Drawing for the job (mm, zero at the part's lowest x, y, z). A direction names the side the tool comes from. Round coordinates to 2 decimals unless told otherwise and drop trailing zeros. Write each loop counter-clockwise with the first axis right and the second up, starting at its lowest first coordinate (ties: lowest second). Pieces come first, ordered by that corner, then holes. Notation, with made-up numbers: (38.5, 85.5) - (75.5, 85.5) arc R11 ccw to (75.5, 95.5) - close; hole circle Ø4 at (89, 39). An arc over 180 degrees is marked (long way). Answer in a Markdown table with one row per item.
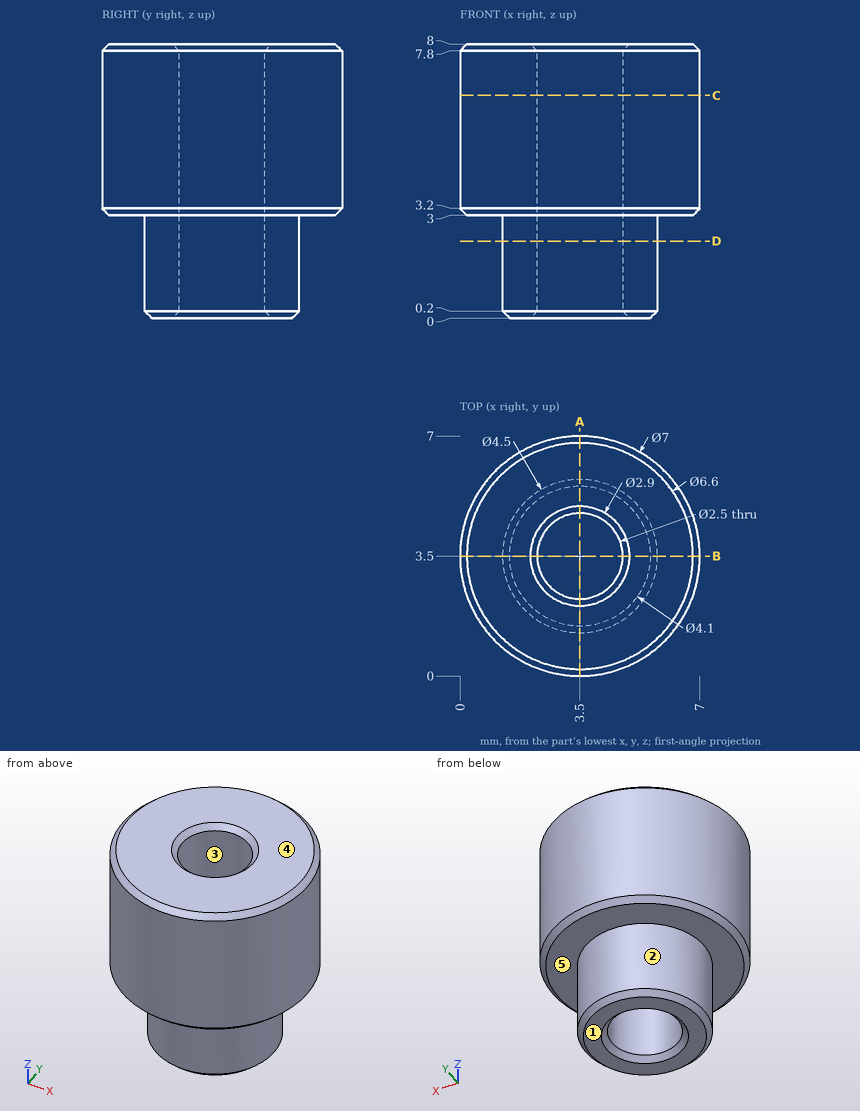
Q1. Saw through at A-A on x = 3.5. List the corners of the cut face in (y, z), then the cut area to 3 significant figures.
Computed:
| item | result |
|---|---|
| outline | (0, 3.2) - (0.2, 3) - (1.25, 3) - (1.25, 0.2) - (1.45, 0) - (2.05, 0) - (2.25, 0.2) - (2.25, 7.8) - (2.05, 8) - (0.2, 8) - (0, 7.8) - close; (4.75, 0.2) - (4.95, 0) - (5.55, 0) - (5.75, 0.2) - (5.75, 3) - (6.8, 3) - (7, 3.2) - (7, 7.8) - (6.8, 8) - (4.95, 8) - (4.75, 7.8) - close |
| area | 28.3 mm2 |
Q2. Drill centre lines: line 1 (Y direction, x = 3.5, z = 6); line 2 (Y direction, x = 3.5, z = 2); line 3 (Z direction, x = 5.75, y = 1.75). Where is each one in solid material? Low to high.
Computed:
| item | result |
|---|---|
| line 1 | y = 0 to 2.25, 4.75 to 7 |
| line 2 | y = 1.25 to 2.25, 4.75 to 5.75 |
| line 3 | z = 3 to 8 |
Q3. Pull direction Y, two halves, no side cores. Call the marked faces 1, 2 and 3: released by +Y, released by -Y, zero draft, split by the parting line, or undercut.
Computed:
| item | result |
|---|---|
| face 1 | zero draft |
| face 2 | split by the parting line |
| face 3 | undercut |
Q4. 3-axis set-ups, long thin cutter, end or side, ignore diameter. For the marked faces 4 and 5: which of +Z, -Z, +X, -X, +Y, -Y reach the whole face in a straight line?
Computed:
| item | result |
|---|---|
| face 4 | +Z, +X, -X, +Y, -Y |
| face 5 | -Z |
Q5. Flat gauge pin, fed straight in: pin 1 (2 mm diameter, centred on y = 5.5, z = 3, fed in from -X). Where does the tip first touch, or does it go through?
Computed:
| item | result |
|---|---|
| pin 1 | stops at x = 0.15 |
Q6. Saw through at C-C on z = 6.5. List the corners of the cut face in (x, y).
Computed:
| item | result |
|---|---|
| outline | circle Ø7 at (3.5, 3.5); hole circle Ø2.5 at (3.5, 3.5) |
Q7. Saw through at D-D on z = 2.25. List the corners of the cut face in (x, y), then the cut area to 3 significant figures.
Computed:
| item | result |
|---|---|
| outline | circle Ø4.5 at (3.5, 3.5); hole circle Ø2.5 at (3.5, 3.5) |
| area | 11.0 mm2 |
